```python
from build123d import *

# Parameters (mm, degrees)
BOSS_EXTRUDE1_DEPTH     = 45
CUT_EXTRUDE1_DEPTH      = 85.483726244
CUT_EXTRUDE1_DEPTH_BACK = 85.483726244
SKETCH3_R               = 10
CUT_EXTRUDE2_DEPTH      = 85.483726244
CUT_EXTRUDE3_DEPTH      = 92.112567739
CUT_EXTRUDE3_DEPTH_BACK = 92.112567739
SKETCH5_W               = 32
SKETCH5_H               = 20
CUT_EXTRUDE4_DEPTH      = 94.441157955
CUT_EXTRUDE4_DEPTH_BACK = 94.441157955
SKETCH4_R               = 6
FILLET1_R               = 3


with BuildPart() as part:
    # Sketch1 → Boss-Extrude1 (new, symmetric)
    with BuildSketch(Plane.XY):
        with BuildLine():
            Line((-30, -12.5), (30, -12.5))
            ThreePointArc((30, -12.5), (42.5, 0), (30, 12.5))
            Line((30, 12.5), (18, 12.5))
            Line((18, 12.5), (18, 22.5))
            Line((18, 22.5), (12, 22.5))
            Line((12, 22.5), (12, 57.5))
            Line((12, 57.5), (-12, 57.5))
            Line((-12, 57.5), (-12, 22.5))
            Line((-12, 22.5), (-18, 22.5))
            Line((-18, 22.5), (-18, 12.5))
            Line((-18, 12.5), (-30, 12.5))
            ThreePointArc((-30, 12.5), (-42.5, 0), (-30, -12.5))
        make_face()
    extrude(amount=BOSS_EXTRUDE1_DEPTH, both=True)

    # Sketch2 → Cut-Extrude1 (cut, two sides: drawn at the far end of the back side and taken through both)
    with BuildSketch(Plane(origin=(0, 0, 0), x_dir=(0, 0, -1), z_dir=(1, 0, 0)).offset(-CUT_EXTRUDE1_DEPTH_BACK)):
        Polygon((-4.585481157, 57.5), (-45, -12.5), (-45, 57.5), align=None)
    extrude(amount=CUT_EXTRUDE1_DEPTH + CUT_EXTRUDE1_DEPTH_BACK, mode=Mode.SUBTRACT)

    # Sketch3 → Cut-Extrude2 (cut, through all)
    with BuildSketch(Plane.XY):
        with Locations(Location((0, 12.5, 0), (0, 0, 90))):
            Circle(SKETCH3_R)
        Polygon((0, 47.5), (-6, 32.5), (6, 32.5), align=None)
    extrude(amount=CUT_EXTRUDE2_DEPTH, mode=Mode.SUBTRACT)

    # Sketch5 → Cut-Extrude3 (cut, two sides: drawn at the far end of the back side and taken through both)
    with BuildSketch(Plane.ZY.offset(12).offset(-CUT_EXTRUDE3_DEPTH_BACK)):
        with Locations((-29, 47.5)):
            Rectangle(SKETCH5_W, SKETCH5_H)
    extrude(amount=CUT_EXTRUDE3_DEPTH + CUT_EXTRUDE3_DEPTH_BACK, mode=Mode.SUBTRACT)

    # Sketch4 → Cut-Extrude4 (cut, two sides: drawn at the far end of the back side and taken through both)
    with BuildSketch(Plane(origin=(0, 57.5, 0), x_dir=(1, 0, 0), z_dir=(0, 1, 0)).offset(-CUT_EXTRUDE4_DEPTH_BACK)):
        with Locations(Location((0, 33, 0), (0, 0, 270))):
            Circle(SKETCH4_R)
    extrude(amount=CUT_EXTRUDE4_DEPTH + CUT_EXTRUDE4_DEPTH_BACK, mode=Mode.SUBTRACT)

    # Fillet1
    fillet1_edges = [part.edges().sort_by_distance(p)[0] for p in [
        (0, 37.5, -45),
        (0, 57.5, -13),
        (0, 37.5, -13),
    ]]
    fillet(fillet1_edges, radius=FILLET1_R)


solid = part.part
```
Check sheet for the modelled part. Datum: model origin and axes. Units: mm. A direction names the side the tool comes from. Give positions to 0.01 mm unless a question says otherwise; leave off trailing zeros. Order: outer loops, then holes, each group sorted by start corner. A loop starts at its lowest first (then second) coordinate and runs counter-clockwise, first axis right, second up. Notation, with made-up numbers: M 23.5,20.5 L 64.5,20.5 A17 cw 64.5,51.5 Z; hole C -13.75,89.5 d8. An arc over 180 degrees is marked long. Answer in a Markdown table with one row per item.
1) Cross-section at C-C, the plane z = -4. Enter the section's corners in (x, y), plus the area to 3 significant figures.
Filled sheet:
| item | result |
|---|---|
| outline | M -30,-12.5 L 30,-12.5 A12.5 ccw 30,12.5 L 18,12.5 L 18,22.5 L 12,22.5 L 12,57.5 L -12,57.5 L -12,22.5 L -18,22.5 L -18,12.5 L -30,12.5 A12.5 ccw Z |
| area | 3,190 mm2 |
2) Cross-section at B-B, the plane x = 2. Enter the section's corners in (y, z), plus the area to 3 significant figures.
Filled sheet:
| item | result |
|---|---|
| outline | M -12.5,-45 L 34.5,-45 A3 ccw 37.5,-42 L 37.5,-38.66 L -12.5,-38.66 Z; M -12.5,-27.34 L 37.5,-27.34 L 37.5,-16 A3 cw 40.5,-13 L 54.5,-13 A3 ccw 57.5,-10 L 57.5,4.59 L 42.5,13.25 L 42.5,0 L 32.5,0 L 32.5,19.02 L 22.3,24.91 L 22.3,0 L 2.7,0 L 2.7,36.22 L -12.5,45 Z |
| area | 2,920 mm2 |
3) Access from +Z, -Z, +X, -X, +Y, -Y to the whole of each face (thin tool, end or side, straight path). Record for faces 4 (the flat face through (24, 12.5, -7)), 5 (the flat face through (0, 38, 0)), 6 (the flat face through (0, 37.5, -26)), 7 (the flat face through (-24, 12.5, -7)).
Filled sheet:
| item | result |
|---|---|
| face 4 | +Z, -Z, +X, +Y |
| face 5 | +Z |
| face 6 | -Z, +X, -X, +Y |
| face 7 | +Z, -Z, -X, +Y |
4) Gauge pin test, flat ends, axial feed: P1, Ø5, axis at x = -15.5, z = 1.5, coming from the +Y side; P2, Ø4, axis at x = -5, y = 44, coming from the -Z side; P3, Ø16, axis at x = 0, y = 16, coming from the +Z side. Record the tip position at first contact, or that the pin passes through.
Filled sheet:
| item | result |
|---|---|
| P1 | stops at y = 22.5 |
| P2 | stops at z = -13 |
| P3 | stops at z = 26.59 |
5) Release check for a two-part mould opening along Y. For faces 1 (the flat face through (-15, 22.5, -10)), 2 (the flat face through (0, 32.5, 9)), 3 (the flat face through (12, 36, -10)) record: +Y half, -Y half, draft (parallel to the pull), parting line (faces both ways), or undercut.
Filled sheet:
| item | result |
|---|---|
| face 1 | +Y half |
| face 2 | undercut |
| face 3 | draft |
6) Thickness scan on L1, parallel to X at y = 14, z = -33; L2, parallel to Y at x = 0, z = 29; L3, parallel to X at y = 10, z = -33. Record the ranges inside material, lowest first. Write a range as [from, to].
Filled sheet:
| item | result |
|---|---|
| L1 | x = [-18, -6], [6, 18] |
| L2 | y = [-12.5, 2.5] |
| L3 | x = [-37.5, -6], [6, 37.5] |
7) Cross-section at A-A, the plane z = -33. Enter the section's corners in (x, y), plus the area to 3 significant figures.
Filled sheet:
| item | result |
|---|---|
| outline | M -30,-12.5 L -6,-12.5 L -6,37.5 L -12,37.5 L -12,22.5 L -18,22.5 L -18,12.5 L -30,12.5 A12.5 ccw Z; M 6,-12.5 L 30,-12.5 A12.5 ccw 30,12.5 L 18,12.5 L 18,22.5 L 12,22.5 L 12,37.5 L 6,37.5 Z |
| area | 2,110 mm2 |
8) Cross-section at D-D, the plane z = 9. Enter the section's corners in (x, y).
Filled sheet:
| item | result |
|---|---|
| outline | M -30,-12.5 L 30,-12.5 A12.5 ccw 30,12.5 L 18,12.5 L 18,22.5 L 12,22.5 L 12,49.85 L -12,49.85 L -12,22.5 L -18,22.5 L -18,12.5 L -30,12.5 A12.5 ccw Z; hole C 0,12.5 d20; hole M -6,32.5 L 6,32.5 L 0,47.5 Z |
